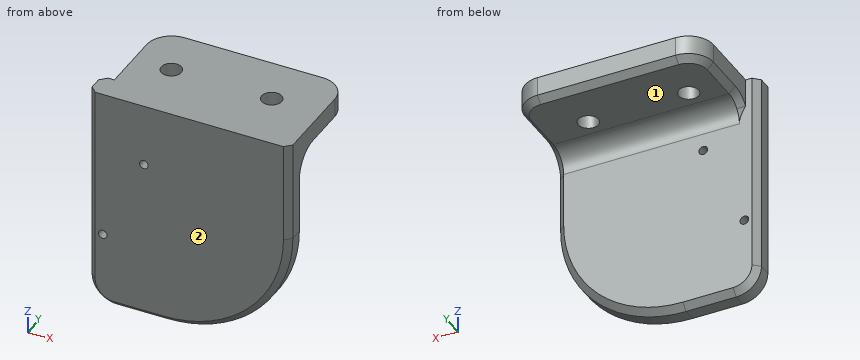
from build123d import *

# Parameters (mm, degrees)
BOSS_EXTRUDE1_DEPTH = 50.8
SKETCH2_R           = 2.54
CUT_EXTRUDE1_DEPTH  = 82.628996839
SKETCH3_R           = 1.0922
CUT_EXTRUDE2_DEPTH  = 82.628996839
FILLET2_R           = 31.75
SKETCH4_W           = 3.175
SKETCH4_H           = 22.225
CUT_EXTRUDE3_DEPTH  = 78.316302453
FILLET3_R           = 6.35
FILLET4_R           = 5.08
CHAMFER1_SIZE       = 1.5875


with BuildPart() as part:
    # Sketch1 → Boss-Extrude1 (new body)
    with BuildSketch(Plane(origin=(0, 0, 0), x_dir=(0, 0, -1), z_dir=(1, 0, 0))):
        Polygon((0, 0), (0, 28.575), (6.35, 28.575), (6.35, 6.35), (57.15, 6.35), (57.15, 0), align=None)
    extrude(amount=BOSS_EXTRUDE1_DEPTH)

    # Sketch2 → Cut-Extrude1 (cut, through all)
    with BuildSketch(Plane.XY):
        with Locations((12.7, 15.875)):
            Circle(SKETCH2_R)
        with Locations(Location((38.1, 15.875, 0), (0, 0, 270))):
            Circle(SKETCH2_R)
    extrude(amount=-CUT_EXTRUDE1_DEPTH, mode=Mode.SUBTRACT)

    # Sketch3 → Cut-Extrude2 (cut, through all)
    with BuildSketch(Plane.XZ):
        with Locations(Location((13.9065, -15.875, 0), (0, 0, 270))):
            Circle(SKETCH3_R)
        with Locations(Location((3.4925, -38.0746, 0), (0, 0, 270))):
            Circle(SKETCH3_R)
    extrude(amount=-CUT_EXTRUDE2_DEPTH, mode=Mode.SUBTRACT)

    # Fillet2
    fillet2_edges = [part.edges().sort_by_distance(p)[0] for p in [
        (50.8, 3.175, -57.15),
    ]]
    fillet(fillet2_edges, radius=FILLET2_R)

    # Sketch4 → Cut-Extrude3 (cut, through all)
    with BuildSketch(Plane(origin=(0, 0, -6.35), x_dir=(-1, 0, 0), z_dir=(0, 0, -1))):
        with Locations((-1.5875, 17.4625)):
            Rectangle(SKETCH4_W, SKETCH4_H)
    extrude(amount=-CUT_EXTRUDE3_DEPTH, mode=Mode.SUBTRACT)

    # Fillet3
    fillet3_edges = [part.edges().sort_by_distance(p)[0] for p in [
        (50.8, 28.575, -3.175),
        (3.175, 28.575, -3.175),
        (0, 3.175, -57.15),
    ]]
    fillet(fillet3_edges, radius=FILLET3_R)

    # Fillet4
    fillet4_edges = [part.edges().sort_by_distance(p)[0] for p in [
        (26.9875, 6.35, -6.35),
    ]]
    fillet(fillet4_edges, radius=FILLET4_R)

    # Chamfer1
    chamfer1_edges = [part.edges().sort_by_distance(p)[0] for p in [
        (50.8, 6.35, -18.415),
        (12.7, 6.35, -57.15),
        (41.500640303, 6.35, -47.850640303),
        (12.7, 0, -57.15),
        (41.500640303, 0, -47.850640303),
        (50.8, 0, -12.7),
        (26.9875, 28.575, -6.35),
        (3.175, 16.8275, -6.35),
        (5.034871939, 26.715128061, -6.35),
        (48.940128061, 26.715128061, -6.35),
        (0, 6.35, -25.4),
        (1.859871939, 6.35, -55.290128061),
        (1.859871939, 0, -55.290128061),
        (50.8, 16.8275, -6.35),
        (3.175, 7.837897552, -7.837897552),
        (50.8, 7.837897552, -7.837897552),
        (0, 0, -25.4),
    ]]
    chamfer(chamfer1_edges, length=CHAMFER1_SIZE)


solid = part.part
CAD build for the part. Positions are in the model's coordinates, mm. Face numbers are marked on the shaded views. A direction names the side the tool comes from. Round coordinates to 2 decimals unless told otherwise and drop trailing zeros.
(1) Drop flat-ended pins along their axis: P1, Ø6.5, axis at x = 38.1, y = 15.875, coming from the -Z side; P2, Ø1, axis at x = 10, z = -18.5, coming from the +Y side; P3, Ø2, axis at x = 24, y = 3, coming from the -Z side. Give the stop position or say it passes through.
(2) Probe line 1 along Y through (x, z) = (12.7, -3.75) (3 decimals); line 2 along Z through (x, y) = (15.5, 21.75); line 3 along Y through (x, z) = (39.5, -40). List the from-to ranges inside material, lowest first.
(3) 3-axis set-ups, long thin cutter, end or side, ignore diameter. For the marked faces 1 and 2: which of +Z, -Z, +X, -X, +Y, -Y reach the whole face in a straight line?
From the geometry:
1. P1: stops at z = -6.35
1. P2: stops at y = 6.35
1. P3: stops at z = -56.9
2. line 1: y = 0 to 13.335, 18.415 to 28.575
2. line 2: z = -6.35 to 0
2. line 3: y = 0 to 6.35
3. face 1: -Z, +X, -X, +Y
3. face 2: +Z, -Z, +X, -X, -Y
